Geometry check sheet. Reference: the model listing, model coordinates, mm. Face numbers are marked on the shaded views. A direction names the side the tool comes from. Round coordinates to 2 decimals unless told otherwise and drop trailing zeros. Write each loop counter-clockwise with the first axis right and the second up, starting at its lowest first coordinate (ties: lowest second). Pieces come first, ordered by that corner, then holes.
Item 1: Scan lines: probe 1 along Z at (x, y) = (4.5, 3); probe 2 along X at (y, z) = (0.25, 7.5); probe 3 along Z at (x, y) = (6.5, -3) (1 decimal). Record each from-to range of solid material in increasing order.
Item 2: Depth check by flat-ended pin: P1, Ø6, axis at x = 5.5, y = 5, coming from the -Z side; P2, Ø1.5, axis at x = 6, z = 1.5, coming from the +Y side. Enter the tip coordinate at first touch or a pass-through.
Item 3: Cross-section at C-C (z = -4). Enter the section's corners in (x, y) (3 decimals), then the cut area to 3 significant figures.
Item 4: Access from +Z, -Z, +X, -X, +Y, -Y to the whole of each face (thin tool, end or side, straight path). Record for the marked faces 3 and 4.
Item 5: Draft check along X on the marked faces 1 and 2. Enter one of: pulls with the +X half, pulls with the -X half, needs draft (parallel to the pull), parting line crosses it, or undercut.
Item 6: Cross-section at D-D (x = -4.25). Enter the section's corners in (y, z) (1 decimal), then the cut area to 3 significant figures.
from build123d import *

# Parameters (mm, degrees)
SKETCH1_R           = 3.175
EXTRUDE1_DEPTH      = 12.7
CHAMFER2_SIZE       = 0.9525
SKETCH27_R          = 6.35
BOSS_EXTRUDE4_DEPTH = 3.175
SKETCH21_R          = 7.9375
BOSS_EXTRUDE1_DEPTH = 7.9375


with BuildPart() as part:
    # Sketch1 → Extrude1 (new body)
    with BuildSketch(Plane.XY):
        Circle(SKETCH1_R)
    extrude(amount=-EXTRUDE1_DEPTH)

    # Chamfer2
    chamfer2_edges = [part.edges().sort_by_distance(p)[0] for p in [
        (-3.175, 0, -12.7),
    ]]
    chamfer(chamfer2_edges, length=CHAMFER2_SIZE)

    # Sketch27 → Boss-Extrude4 (add)
    with BuildSketch(Plane.XY):
        Circle(SKETCH27_R)
    extrude(amount=BOSS_EXTRUDE4_DEPTH)

    # Sketch21 → Boss-Extrude1 (add)
    with BuildSketch(Plane.XY.offset(3.175)):
        Circle(SKETCH21_R)
    extrude(amount=BOSS_EXTRUDE1_DEPTH)


solid = part.part
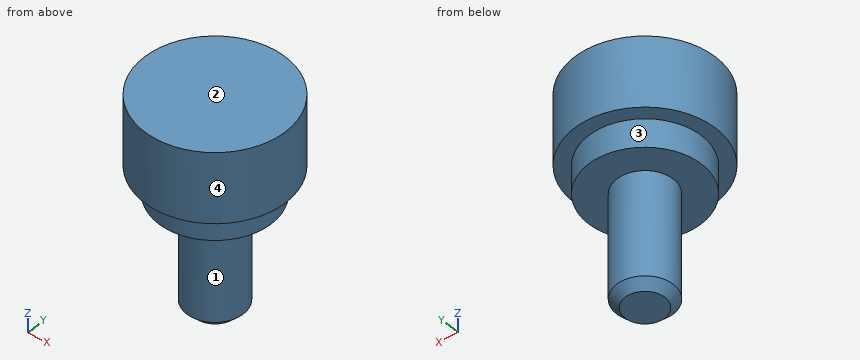
Resolved:
1. probe 1: z = 0 to 11.11
1. probe 2: x = -7.93 to 7.93
1. probe 3: z = 3.2 to 11.1
2. P1: stops at z = 0
2. P2: stops at y = 3.57
3. outline: circle Ø6.35 at (0, 0)
3. area: 31.7 mm2
4. face 3: -Z
4. face 4: +Z, -Z
5. face 1: parting line crosses it
5. face 2: needs draft
6. outline: (-6.7, 3.2) - (-4.7, 3.2) - (-4.7, 0) - (4.7, 0) - (4.7, 3.2) - (6.7, 3.2) - (6.7, 11.1) - (-6.7, 11.1) - close
6. area: 136 mm2
